```python
from build123d import *

# Parameters (mm, degrees)
SKETCH_1_R               = 6
EXTRUDE_1_DEPTH          = 8
SKETCH_2_W               = 5.05
SKETCH_2_H               = 1.88
SKETCH_2_W_2             = 1.88
SKETCH_2_H_2             = 5.15
CUT_EXTRUDE_1_DEPTH      = 12.66190379
FILLET_1_R               = 0.6
CUT_EXTRUDE_2_DEPTH      = 0.5
CUT_EXTRUDE_2_DEPTH_BACK = 14.17310233
SKETCH_3_R               = 1.2


with BuildPart() as part:
    # ｽｹｯﾁ1 → ﾎﾞｽ - 押し出し1 (new body)
    with BuildSketch(Plane.XY):
        Circle(SKETCH_1_R)
    extrude(amount=EXTRUDE_1_DEPTH)

    # ｽｹｯﾁ2 → ｶｯﾄ - 押し出し1 (cut, through all)
    with BuildSketch(Plane.XY.offset(8)):
        Rectangle(SKETCH_2_W, SKETCH_2_H)
        Rectangle(SKETCH_2_W_2, SKETCH_2_H_2)
    extrude(amount=-CUT_EXTRUDE_1_DEPTH, mode=Mode.SUBTRACT)

    # ﾌｨﾚｯﾄ1
    fillet_1_edges = [part.edges().sort_by_distance(p)[0] for p in [
        (-0.94, 0.94, 4),
        (0.94, -0.94, 4),
        (-0.94, -0.94, 4),
        (0.94, 0.94, 4),
    ]]
    fillet(fillet_1_edges, radius=FILLET_1_R)

    # ｽｹｯﾁ3 → ｶｯﾄ - 押し出し2 (cut, two sides: drawn at the far end of the back side and taken through both)
    with BuildSketch(Plane(origin=(0, -2.575, 0), x_dir=(1, 0, 0), z_dir=(0, 1, 0)).offset(-CUT_EXTRUDE_2_DEPTH_BACK)):
        with Locations(Location((0, -4, 0), (0, 0, 90))):
            Circle(SKETCH_3_R)
    extrude(amount=CUT_EXTRUDE_2_DEPTH + CUT_EXTRUDE_2_DEPTH_BACK, mode=Mode.SUBTRACT)


solid = part.part
```
Build history of the part. All positions in model axes, mm. A direction names the side the tool comes from. Coordinates: 2 decimals unless noted, no trailing zeros. Order: outer loops, then holes, each group sorted by start corner. A loop starts at its lowest first (then second) coordinate and runs counter-clockwise, first axis right, second up. Notation, with made-up numbers: M 21,41.5 L 42,41.5 A12 cw 42,63.5 Z; hole C -40,41 d11. An arc over 180 degrees is marked long. One line per question, with ' | ' between items. Start each with the question number.
1. Tool access for faces 1 (the face through (-0.36, -4.067, 2.855)), 2 (the face through (1.25, -1.25, 8)), 3 (the face through (0, 2.575, 4)): list every direction of +Z, -Z, +X, -X, +Y, -Y with a clear straight run to the whole face (end or side of a thin tool).
2. Mould opens along X. For faces 4 (the face through (-0.94, 2, 4)), 5 (the face through (2.525, 0, 4)), 6 (the face through (-6, 0, 4)), 7 (the face through (1.25, -1.25, 0)) say: +X half, -X half, draft (parallel to the pull), parting line (faces both ways), or undercut.
3. Cut at A-A (x = 0). Write the cut outline in (y, z) (3 decimals).
4. Cut at C-C (z = 2). Write the cut outline in (x, y) (3 decimals), plus the area to 3 significant figures.
5. Wall check: line 1 along Y through (x, z) = (0, 7.25) (3 decimals); line 2 along X through (y, z) = (-1, 3); line 3 along Y through (x, z) = (1.25, 4). Give the ranges that are in metal, low to high. Write a range as [from, to].
6. Cut at B-B (y = 0). Write the cut outline in (x, z) (3 decimals).
7. Cut at D-D (y = -4). Write the cut outline in (x, z), plus the area to 3 significant figures.
8. Flat gauge pins, fed straight in: P1, Ø0.8, axis at y = -2, z = 5, coming from the +X side; P2, Ø1.1, axis at x = -2, z = 6, coming from the -Y side; P3, Ø0.5, axis at y = -2, z = 2, coming from the -X side. Where does each tip first touch, or does it go through?
The answers:
1) face 1: -Y | face 2: +Z, +X, -X, +Y, -Y | face 3: +Z, -Z
2) face 4: undercut | face 5: undercut | face 6: parting line | face 7: draft
3) outline: M -6,0 L -2.575,0 L -2.575,2.8 L -6,2.8 Z; M -6,5.2 L -2.575,5.2 L -2.575,8 L -6,8 Z; M 2.575,0 L 6,0 L 6,8 L 2.575,8 Z
4) outline: C 0,0 d12; hole M -2.525,-0.94 L -1.54,-0.94 A0.6 cw -0.94,-1.54 L -0.94,-2.575 L 0.94,-2.575 L 0.94,-1.54 A0.6 cw 1.54,-0.94 L 2.525,-0.94 L 2.525,0.94 L 1.54,0.94 A0.6 cw 0.94,1.54 L 0.94,2.575 L -0.94,2.575 L -0.94,1.54 A0.6 cw -1.54,0.94 L -2.525,0.94 Z | area: 97.1 mm2
5) line 1: y = [-6, -2.575], [2.575, 6] | line 2: x = [-5.92, -1.28], [1.28, 5.92] | line 3: y = [-5.87, -1.01], [1.01, 5.87]
6) outline: M -6,0 L -2.525,0 L -2.525,8 L -6,8 Z; M 2.525,0 L 6,0 L 6,8 L 2.525,8 Z
7) outline: M -4.47,0 L 4.47,0 L 4.47,8 L -4.47,8 Z; hole C 0,4 d2.4 | area: 67.0 mm2
8) P1: stops at x = 5.78 | P2: stops at y = -5.82 | P3: stops at x = -5.74
